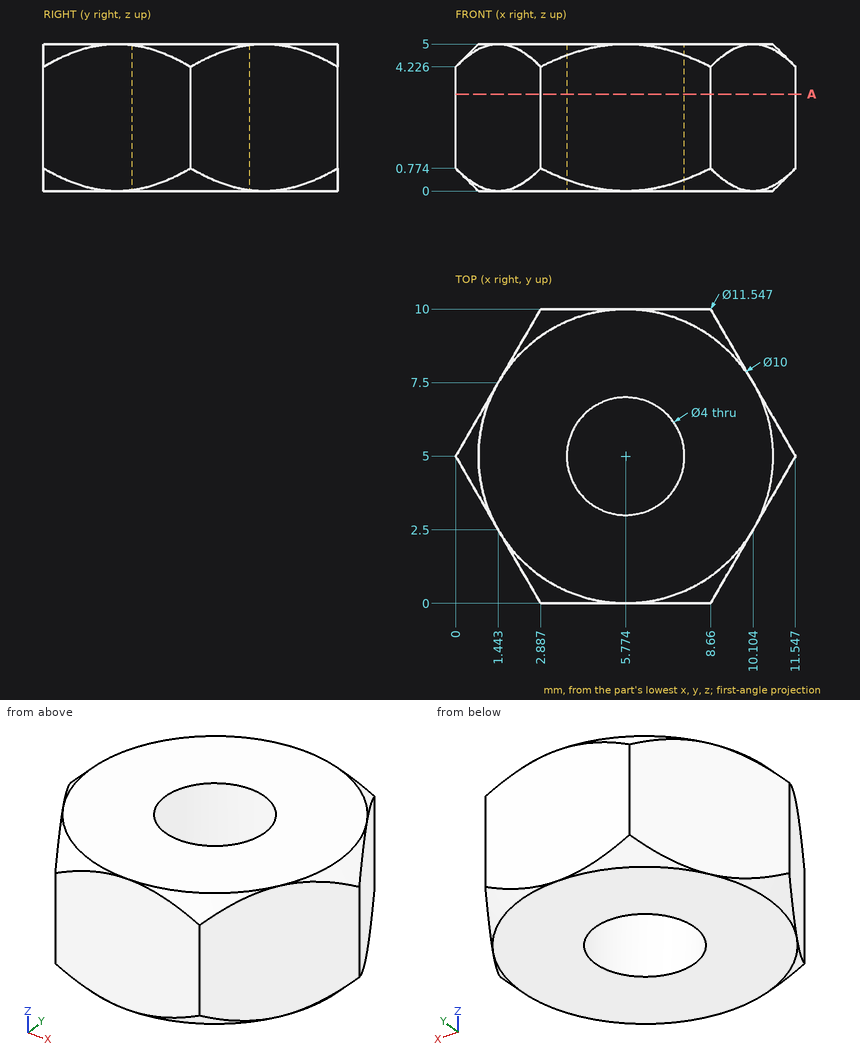
Geometry check sheet. Reference: drawing and pictorial views, mm from the part's lowest x, y, z. Give positions to 0.01 mm unless a question says otherwise; leave off trailing zeros. Order: outer loops, then holes, each group sorted by start corner. A loop starts at its lowest first (then second) coordinate and runs counter-clockwise, first axis right, second up. Notation, with made-up numbers: M -36.75,8.25 L -19.75,8.25 A15 ccw -19.75,19.25 Z; hole C 82,-12 d9. An arc over 180 degrees is marked long. Answer in a Markdown table with one row per item. Add a question column.
Q1. Gauge pin test, flat ends, axial feed: pin 1 Ø3 at (y, z) = (7, 3) entering from -X; pin 2 Ø1.5 at (x, z) = (9.5, 0.5) entering from -Y; pin 3 Ø1 at (x, z) = (1.5, 4) entering from +Y (1 decimal); pin 4 Ø5 at (x, y) = (5.77, 5) entering from -Z. Record the tip position at first contact, or that the pin passes through.
Q2. Thickness scan on L1, parallel to Y at x = 5.75, z = 1.9; L2, parallel to Y at x = 6.5, z = 1.1 (1 decimal); L3, parallel to X at y = 7.5, z = 2.45 (1 decimal). Record the ranges inside material, lowest first.
Q3. Sectioned sample at A-A, the plane z = 3.3. Record the boundary of the cut face in (x, y).
Verdict:
| question | item | result |
|---|---|---|
| 1 | pin 1 | x = 0.29 |
| 1 | pin 2 | y = 0.19 |
| 1 | pin 3 | y = 8.5 |
| 1 | pin 4 | z = 0 |
| 2 | L1 | 0 to 3, 7 to 10 |
| 2 | L2 | 0 to 3.1, 6.9 to 10 |
| 2 | L3 | 1.4 to 10.1 |
| 3 | outline | M 0,5 L 2.89,0 L 8.66,0 L 11.55,5 L 8.66,10 L 2.89,10 Z; hole C 5.77,5 d4 |
